from build123d import *

# Parameters (mm, degrees)
F0_W      = 5.08
F0_H      = 1.27
F0_W_2    = 1.27
F0_H_2    = 5.08
F1_DEPTH  = 12.7
F3_FACE_R = 15.875
F4_DEPTH  = 1.27


with BuildPart() as f1:
    # F0 (on Front) → F1 (new body)
    with BuildSketch(Plane.XZ):
        with Locations((0, 8.545089)):
            Rectangle(F0_W, F0_H)
        with BuildLine():
            Line((-2.54, 9.180089), (2.54, 9.180089))
            ThreePointArc((2.54, 9.180089), (0, 9.525), (-2.54, 9.180089))
        make_face()
        with Locations((-8.545089, 0)):
            Rectangle(F0_W_2, F0_H_2)
        with BuildLine():
            Line((-9.180089, -2.54), (-9.180089, 2.54))
            ThreePointArc((-9.180089, 2.54), (-9.525, 0), (-9.180089, -2.54))
        make_face()
        with BuildLine():
            ThreePointArc((-2.54, -9.180089), (0, -9.525), (2.54, -9.180089))
            Line((2.54, -9.180089), (-2.54, -9.180089))
        make_face()
        with Locations((0, -8.545089)):
            Rectangle(F0_W, F0_H)
        with Locations((8.545089, 0)):
            Rectangle(F0_W_2, F0_H_2)
        with BuildLine():
            ThreePointArc((9.180089, -2.54), (9.438378, -1.281656), (9.525, 0))
            ThreePointArc((9.525, 0), (9.438378, 1.281656), (9.180089, 2.54))
            Line((9.180089, 2.54), (9.180089, -2.54))
        make_face()
    extrude(amount=F1_DEPTH)

    # F2 (on Right) → F3 (revolve)
    with BuildSketch(Plane.YZ):
        with BuildLine():
            Line((0, 15.875), (0, 0))
            Line((0, 0), (5.08, 0))
            ThreePointArc((5.08, 0), (3.790842, 8.33777), (0, 15.875))
        make_face()
    revolve(axis=Axis((0, 2.54, 0), (0, 1, 0)))

    # F3_face (on face) → F4 (join)
    with BuildSketch(Plane.XZ):
        Circle(F3_FACE_R)
        with BuildLine():
            Line((-7.910089, 2.54), (-7.910089, -2.54))
            Line((-7.910089, -2.54), (-9.180089, -2.54))
            ThreePointArc((-9.180089, -2.54), (-9.525, 0), (-9.180089, 2.54))
            Line((-9.180089, 2.54), (-7.910089, 2.54))
        make_face(mode=Mode.SUBTRACT)
        with BuildLine():
            Line((-2.54, -9.180089), (-2.54, -7.910089))
            Line((-2.54, -7.910089), (2.54, -7.910089))
            Line((2.54, -7.910089), (2.54, -9.180089))
            ThreePointArc((2.54, -9.180089), (0, -9.525), (-2.54, -9.180089))
        make_face(mode=Mode.SUBTRACT)
        with BuildLine():
            Line((2.54, 7.910089), (-2.54, 7.910089))
            Line((-2.54, 7.910089), (-2.54, 9.180089))
            ThreePointArc((-2.54, 9.180089), (0, 9.525), (2.54, 9.180089))
            Line((2.54, 9.180089), (2.54, 7.910089))
        make_face(mode=Mode.SUBTRACT)
        with BuildLine():
            ThreePointArc((9.180089, 2.54), (9.525, 0), (9.180089, -2.54))
            Line((9.180089, -2.54), (7.910089, -2.54))
            Line((7.910089, -2.54), (7.910089, 2.54))
            Line((7.910089, 2.54), (9.180089, 2.54))
        make_face(mode=Mode.SUBTRACT)
    extrude(amount=F4_DEPTH)


solid = f1.part
Geometry check sheet. Reference: the model listing, model coordinates, mm. A direction names the side the tool comes from. Give positions to 0.01 mm unless a question says otherwise; leave off trailing zeros. Order: outer loops, then holes, each group sorted by start corner. A loop starts at its lowest first (then second) coordinate and runs counter-clockwise, first axis right, second up.
1. Draft check along Z on faces 5 (the face through (-9, -7, 2.54)), 6 (the face through (0, -12.7, 9)), 7 (the face through (0, -7, 7.91)), 8 (the face through (-9, -7, -2.54)). Enter one of: pulls with the +Z half, pulls with the -Z half, needs draft (parallel to the pull), parting line crosses it, or undercut.
Completed:
face 5: pulls with the +Z half
face 6: needs draft
face 7: undercut
face 8: pulls with the -Z half
2. Depth check by flat-ended pin: pin 1 (1.5 mm diameter, centred on x = 0.5, z = -2, fed in from +Y); pin 2 (0.6 mm diameter, centred on x = -8.5, y = -4.5, fed in from -Z); pin 3 (8 mm diameter, centred on x = 1, y = -2, fed in from +Z) (3 decimals); pin 4 (0.6 mm diameter, centred on x = 9, y = -6.5, fed in from +Z). Enter the tip coordinate at first touch or a pass-through.
Completed:
pin 1: stops at y = 5.05
pin 2: stops at z = -2.54
pin 3: stops at z = 15.875
pin 4: stops at z = 2.54
3. Scan lines: line 1 (Z direction, x = 2.5, y = -6.5); line 2 (X direction, y = -9.75, z = -9); line 3 (Y direction, x = 3.5, z = 11). Record each from-to range of solid material in increasing order.
Completed:
line 1: z = -9.19 to -7.91, 7.91 to 9.19
line 2: x = -2.54 to 2.54
line 3: y = -1.27 to 2.54
4. Sectioned sample at A-A (y = -3). Record the boundary of the cut face in (x, z) (3 decimals).
Completed:
outline: (-9.18, -2.54) - (-7.91, -2.54) - (-7.91, 2.54) - (-9.18, 2.54) arc R9.525 ccw to start; (-2.54, -9.18) arc R9.525 ccw to (2.54, -9.18) - (2.54, -7.91) - (-2.54, -7.91) - close; (-2.54, 7.91) - (2.54, 7.91) - (2.54, 9.18) arc R9.525 ccw to (-2.54, 9.18) - close; (7.91, -2.54) - (9.18, -2.54) arc R9.525 ccw to (9.525, 0) arc R9.525 ccw to (9.18, 2.54) - (7.91, 2.54) - close
5. Access from +Z, -Z, +X, -X, +Y, -Y to the whole of each face (thin tool, end or side, straight path). Record for faces 1 (the face through (-9.525, -6.905, 0.036)), 2 (the face through (-2.54, -7, 9)), 3 (the face through (0, -7, -7.91)), 4 (the face through (-7.91, -7, 0)).
Completed:
face 1: -X, -Y
face 2: +Z, -Z, -X, -Y
face 3: +X, -X, -Y
face 4: +Z, -Z, -Y
